from build123d import *

# Parameters (mm, degrees)
F2_R      = 3.05
F3_DEPTH  = 15
F4_R      = 0.5
F5_R      = 1.2
F6_DEPTH  = 7
F7_R      = 1.5
F8_DEPTH  = 15
F9_R      = 3.55
F10_DEPTH = 2
F11_R     = 2.5
F12_DEPTH = 3


with BuildPart() as f1:
    # F0 (on Front) → F1 (revolve)
    with BuildSketch(Plane.XZ):
        Polygon((-5, 0), (0, 0), (0, 17), (-6.5, 17), (-6.5, 0), align=None)
    revolve(axis=Axis((0, 0, -3.667768), (0, 0, -1)))

    # F2 (on face) → F3 (cut)
    with BuildSketch(Plane(origin=(0, 0, 0), x_dir=(1, 0, 0), z_dir=(0, 0, -1))):
        Circle(F2_R)
    extrude(amount=-F3_DEPTH, mode=Mode.SUBTRACT)

    # F4
    f4_edges = [f1.edges().sort_by_distance(p)[0] for p in [
        (6.5, 0, 17),
    ]]
    fillet(f4_edges, radius=F4_R)

    # F5 (on Front) → F6 (cut)
    with BuildSketch(Plane.XZ):
        with Locations((0, 11)):
            Circle(F5_R)
    extrude(amount=F6_DEPTH, mode=Mode.SUBTRACT)

    # F7 (on face) → F8 (cut)
    with BuildSketch(Plane(origin=(0, 0, 0), x_dir=(1, 0, 0), z_dir=(0, 0, -1))):
        with Locations((-7.5, 0)):
            Circle(F7_R)
        with Locations((-6.495191, -3.75)):
            Circle(F7_R)
        with Locations((-3.75, -6.495191)):
            Circle(F7_R)
        with Locations((0, -7.5)):
            Circle(F7_R)
        with Locations((3.75, -6.495191)):
            Circle(F7_R)
        with Locations((6.495191, -3.75)):
            Circle(F7_R)
        with Locations((7.5, 0)):
            Circle(F7_R)
        with Locations((6.495191, 3.75)):
            Circle(F7_R)
        with Locations((3.75, 6.495191)):
            Circle(F7_R)
        with Locations((0, 7.5)):
            Circle(F7_R)
        with Locations((-3.75, 6.495191)):
            Circle(F7_R)
        with Locations((-6.495191, 3.75)):
            Circle(F7_R)
    extrude(amount=-F8_DEPTH, mode=Mode.SUBTRACT)

    # F9 (on face) → F10 (cut)
    with BuildSketch(Plane(origin=(0, 0, 0), x_dir=(1, 0, 0), z_dir=(0, 0, -1))):
        Circle(F9_R)
    extrude(amount=-F10_DEPTH, mode=Mode.SUBTRACT)

    # F11 (on face) → F12 (cut)
    with BuildSketch(Plane.XY.offset(17)):
        Circle(F11_R)
    extrude(amount=-F12_DEPTH, mode=Mode.SUBTRACT)


solid = f1.part
The listing builds one solid part. Answer for the finished solid, in the listing's coordinates (mm). A direction names the side the tool comes from. Coordinates: 2 decimals unless noted, no trailing zeros. Loops run counter-clockwise (first coordinate to the right, second up) from the corner with the lowest first, then second, coordinate; pieces in that order, holes last. Notation, with made-up numbers: M -22,-21 L -1,-21 A33 ccw -1,11 Z; hole C -9.5,87 d6. An arc over 180 degrees is marked long. Answer in a Markdown table with one row per item.
1) Find section D-D (z = 11). Determine the outline of the cut face in (x, y).
Answers below:
| item | result |
|---|---|
| outline | M -6.42,-1.04 A6.5 ccw -6.08,-2.31 A1.5 cw -5.04,-4.11 A6.5 ccw -4.11,-5.04 A1.5 cw -2.31,-6.08 A6.5 ccw -1.2,-6.39 L -1.2,-2.8 A3.05 cw long 1.2,-2.8 L 1.2,-6.39 A6.5 ccw 2.31,-6.08 A1.5 cw 4.11,-5.04 A6.5 ccw 5.04,-4.11 A1.5 cw 6.08,-2.31 A6.5 ccw 6.42,-1.04 A1.5 cw 6.42,1.04 A6.5 ccw 6.08,2.31 A1.5 cw 5.04,4.11 A6.5 ccw 4.11,5.04 A1.5 cw 2.31,6.08 A6.5 ccw 1.04,6.42 A1.5 cw -1.04,6.42 A6.5 ccw -2.31,6.08 A1.5 cw -4.11,5.04 A6.5 ccw -5.04,4.11 A1.5 cw -6.08,2.31 A6.5 ccw -6.42,1.04 A1.5 cw Z |
2) Determine the mould class of faces 5 (the cylindrical face through (-1.2, -4.59, 11.05)), 6 (the cylindrical face through (-5.19, 3.01, 7.4)), 7 (the cylindrical face through (6, 0, 7)), 8 (the flat face through (-5.4, 3.1, 15)) for opening direction X: released by +X, released by -X, zero draft, split by the parting line, or undercut.
Answers below:
| item | result |
|---|---|
| face 5 | undercut |
| face 6 | released by -X |
| face 7 | released by +X |
| face 8 | zero draft |
3) Find section A-A (y = 0). Determine the outline of the cut face in (x, z).
Answers below:
| item | result |
|---|---|
| outline | M -6.5,15 L -6,15 L -6,0 L -3.55,0 L -3.55,2 L -3.05,2 L -3.05,15 L -2.5,15 L -2.5,17 L -6,17 A0.5 ccw -6.5,16.5 Z; M 2.5,15 L 3.05,15 L 3.05,2 L 3.55,2 L 3.55,0 L 6,0 L 6,15 L 6.5,15 L 6.5,16.5 A0.5 ccw 6,17 L 2.5,17 Z |
4) Find section B-B (x = 0). Determine the outline of the cut face in (y, z), then the cut area to 3 significant figures.
Answers below:
| item | result |
|---|---|
| outline | M -6.5,15 L -6,15 L -6,12.2 L -3.05,12.2 L -3.05,15 L -2.5,15 L -2.5,17 L -6,17 A0.5 ccw -6.5,16.5 Z; M -6,0 L -3.55,0 L -3.55,2 L -3.05,2 L -3.05,9.8 L -6,9.8 Z; M 2.5,15 L 3.05,15 L 3.05,2 L 3.55,2 L 3.55,0 L 6,0 L 6,15 L 6.5,15 L 6.5,16.5 A0.5 ccw 6,17 L 2.5,17 Z |
| area | 95.3 mm^2 |
5) Find the intervals of material crossed by probe 1 along X at (y, z) = (0, 9.75); probe 2 along X at (y, z) = (0, 0.9), in increasing order.
Answers below:
| item | result |
|---|---|
| probe 1 | -6 to -3.05, 3.05 to 6 |
| probe 2 | -6 to -3.55, 3.55 to 6 |
6) Which of the six approach directions +Z, -Z, +X, -X, +Y, -Y give full straight-line access (tool end or side, diameter ignored) to faces 1 (the cylindrical face through (-0.661, 2.977, 8.409)), 2 (the cylindrical face through (0, -6, 5)), 3 (the cylindrical face through (3.01, 5.19, 7.4)), 4 (the cylindrical face through (-5.2, -2.99, 7.4))?
Answers below:
| item | result |
|---|---|
| face 1 | -Z |
| face 2 | -Z, -Y |
| face 3 | -Z, +Y |
| face 4 | -Z, -X |
7) Given pin 1 (2 mm diameter, centred on y = -4, z = 4.5, fed in from +X); pin 2 (3 mm diameter, centred on x = 1, y = -0.5, fed in from -Z); pin 3 (5 mm diameter, centred on y = 5, z = 13.5, fed in from -X); pin 4 (2 mm diameter, centred on x = 0.5, y = -1, fed in from -Z), each flat-ended and moving along its own axis, determine where each tip first touches the part or whether it passes through.
Answers below:
| item | result |
|---|---|
| pin 1 | x = 5.2 |
| pin 2 | z = 15 |
| pin 3 | x = -5.77 |
| pin 4 | through |
8) Find section C-C (z = 16). Determine the outline of the cut face in (x, y), then the cut area to 3 significant figures.
Answers below:
| item | result |
|---|---|
| outline | C 0,0 d13; hole C 0,0 d5 |
| area | 113 mm^2 |
